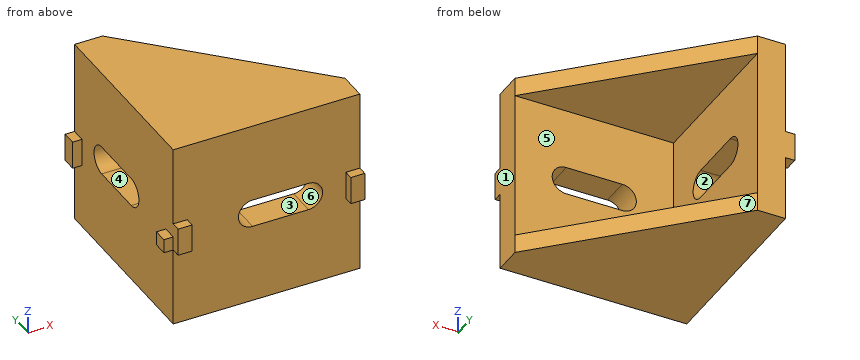
```python
from build123d import *

# Parameters (mm, degrees)
SALIENTE_EXTRUIR1_DEPTH = 20
SALIENTE_EXTRUIR2_DEPTH = 2
SALIENTE_EXTRUIR3_DEPTH = 2
CORTAR_EXTRUIR1_DEPTH   = 4
CORTAR_EXTRUIR2_DEPTH   = 4
CROQUIS6_W              = 1.5
CROQUIS6_H              = 3
SALIENTE_EXTRUIR4_DEPTH = 1
CROQUIS7_W              = 3
CROQUIS7_H              = 1.5
CROQUIS7_W_2            = 1.5
SALIENTE_EXTRUIR6_DEPTH = 1


with BuildPart() as part:
    # Croquis1 → Saliente-Extruir1 (new body)
    with BuildSketch(Plane.XY):
        Polygon((0, 20), (3, 20), (3, 3), (20, 3), (20, 0), (0, 0), align=None)
    extrude(amount=SALIENTE_EXTRUIR1_DEPTH)

    # Croquis2 → Saliente-Extruir2 (add)
    with BuildSketch(Plane.XY.offset(20)):
        Polygon((3, 20), (20, 3), (20, 0), (0, 0), (0, 20), align=None)
    extrude(amount=-SALIENTE_EXTRUIR2_DEPTH)

    # Croquis3 → Saliente-Extruir3 (add)
    with BuildSketch(Plane(origin=(0, 0, 0), x_dir=(-1, 0, 0), z_dir=(0, 0, -1))):
        Polygon((0, 20), (-3, 20), (-20, 3), (-20, 0), (0, 0), align=None)
    extrude(amount=-SALIENTE_EXTRUIR3_DEPTH)

    # Croquis4 → Cortar-Extruir1 (cut, through all)
    with BuildSketch(Plane(origin=(3, 0, 0), x_dir=(0, 0, -1), z_dir=(1, 0, 0))):
        with BuildLine():
            Line((-11.54072, 8.5), (-11.54072, 14.5))
            ThreePointArc((-11.54072, 14.5), (-10, 16.04072), (-8.45928, 14.5))
            Line((-8.45928, 14.5), (-8.45928, 8.5))
            ThreePointArc((-8.45928, 8.5), (-10, 6.95928), (-11.54072, 8.5))
        make_face()
    extrude(amount=-CORTAR_EXTRUIR1_DEPTH, mode=Mode.SUBTRACT)

    # Croquis5 → Cortar-Extruir2 (cut, through all)
    with BuildSketch(Plane(origin=(0, 3, 0), x_dir=(1, 0, 0), z_dir=(0, 1, 0))):
        with BuildLine():
            Line((8.5, -8.492105493), (14.5, -8.492105493))
            ThreePointArc((14.5, -8.492105493), (16.007894507, -10), (14.5, -11.507894507))
            Line((14.5, -11.507894507), (8.5, -11.507894507))
            ThreePointArc((8.5, -11.507894507), (6.992105493, -10), (8.5, -8.492105493))
        make_face()
    extrude(amount=-CORTAR_EXTRUIR2_DEPTH, mode=Mode.SUBTRACT)

    # Croquis6 → Saliente-Extruir4 (add)
    with BuildSketch(Plane.XZ):
        with Locations((0.75, 10)):
            Rectangle(CROQUIS6_W, CROQUIS6_H)
        with Locations((19.25, 10)):
            Rectangle(CROQUIS6_W, CROQUIS6_H)
    extrude(amount=SALIENTE_EXTRUIR4_DEPTH)

    # Croquis7 → Saliente-Extruir6 (add)
    with BuildSketch(Plane.ZY):
        with Locations((8.5, 19.25)):
            Rectangle(CROQUIS7_W, CROQUIS7_H)
        with Locations((9.25, 0.75)):
            Rectangle(CROQUIS7_W_2, CROQUIS7_H)
    extrude(amount=SALIENTE_EXTRUIR6_DEPTH)


solid = part.part
```
The listing builds one solid part. Answer for the finished solid, in the listing's coordinates (mm). Face numbers are marked on the shaded views. A direction names the side the tool comes from. Coordinates: 2 decimals unless noted, no trailing zeros. Loops run counter-clockwise (first coordinate to the right, second up) from the corner with the lowest first, then second, coordinate; pieces in that order, holes last. Notation, with made-up numbers: M 55,30 L 100,30 A10 cw 100,40 Z; hole C 9,-38.5 d11. An arc over 180 degrees is marked long. Answer as CSV lines item,"result". Start each with the question number.
(1) The part is cut by section D-D (x = 15.25). Give the vertices of the cut face in (y, z), and give its area (3 significant figures).
(2) The mould has two halves that part along X. Classify the marked faces 1, 2 and 3: pulls with the +X half, pulls with the -X half, needs draft (parallel to the pull), parting line crosses it, or undercut.
(3) The part is cut by section C-C (z = 2.5). Give the vertices of the cut face in (x, y).
(4) Given pin 1 (0.5 mm diameter, centred on y = -0.5, z = 9.5, fed in from -X); pin 2 (2 mm diameter, centred on y = 6, z = 14, fed in from +X); pin 3 (5 mm diameter, centred on x = 14, z = 11.5, fed in from +Y), each flat-ended and moving along its own axis, determine where each tip first touches the part or whether it passes through.
(5) Find the intervals of material crossed by L1, parallel to Z at x = 7.5, y = 4.5; L2, parallel to Y at x = 19.25, z = 12.75; L3, parallel to X at y = 1, z = 1, in increasing order. Write a range as [from, to].
(6) For the marked faces 4, 5, 6 and 7, determine the directions among +Z, -Z, +X, -X, +Y, -Y from which every point of the face is accessible in a straight line to the end or side of a thin tool.
(7) The part is cut by section B-B (y = 0.75). Give the vertices of the cut face in (x, z).
(8) The part is cut by section A-A (y = 13.5). Give the vertices of the cut face in (x, z), and give its area (3 significant figures).
Determined:
1,outline,"M 0,0 L 7.75,0 L 7.75,2 L 3,2 L 3,8.69 L 0,8.69 Z; M 0,11.31 L 3,11.31 L 3,18 L 7.75,18 L 7.75,20 L 0,20 Z"
1,area,"71.2 mm2"
2,face 1,"pulls with the +X half"
2,face 2,"needs draft"
2,face 3,"undercut"
3,outline,"M 0,0 L 20,0 L 20,3 L 3,3 L 3,20 L 0,20 Z"
4,pin 1,"x = 0"
4,pin 2,"x = 3"
4,pin 3,"y = 3"
5,L1,"[0, 2], [18, 20]"
5,L2,"[0, 3]"
5,L3,"[0, 20]"
6,face 4,"+X, -X"
6,face 5,"+X, +Y"
6,face 6,"+Y, -Y"
6,face 7,"+Z, -Z, +X, +Y"
7,outline,"M -1,8.5 L 0,8.5 L 0,0 L 20,0 L 20,20 L 0,20 L 0,10 L -1,10 Z; hole M 8.5,8.49 L 14.5,8.49 A1.51 ccw 14.5,11.51 L 8.5,11.51 A1.51 ccw Z"
8,outline,"M 0,0 L 9.5,0 L 9.5,2 L 3,2 L 3,8.46 L 0,8.46 Z; M 0,11.54 L 3,11.54 L 3,18 L 9.5,18 L 9.5,20 L 0,20 Z"
8,area,"76.8 mm2"
